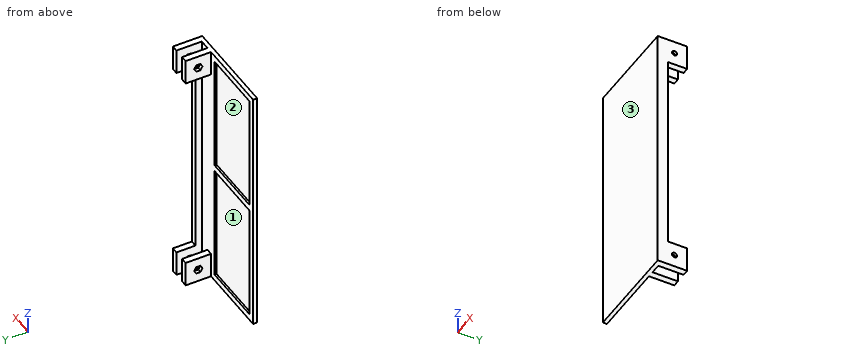
from build123d import *

# Parameters (mm, degrees)
F0_W      = 60
F0_H      = 200
F1_DEPTH  = 3.2
F2_W      = 3
F2_H      = 20
F3_DEPTH  = 20
F5_DEPTH  = 15
F6_DEPTH  = 2
F7_DEPTH  = 2
F8_R      = 2
F9_DEPTH  = 3
F10_DEPTH = 25
F11_R     = 2
F12_DEPTH = 3
F13_DEPTH = 25
F14_W     = 5
F14_H     = 5
F15_DEPTH = 160
F16_W     = 49
F16_H     = 92.5
F17_DEPTH = 1.6


with BuildPart() as f1:
    # F0 (on Front) → F1 (new body)
    with BuildSketch(Plane.XZ):
        with Locations((30, 100)):
            Rectangle(F0_W, F0_H)
    extrude(amount=F1_DEPTH)

    # F2 (on face) → F3 (join)
    with BuildSketch(Plane(origin=(0, 0, 0), x_dir=(-1, 0, 0), z_dir=(0, 1, 0))):
        with Locations((-58.5, 190)):
            Rectangle(F2_W, F2_H)
        with Locations((-58.5, 10)):
            Rectangle(F2_W, F2_H)
        with Locations((-47.5, 190)):
            Rectangle(F2_W, F2_H)
        with Locations((-47.5, 10)):
            Rectangle(F2_W, F2_H)
    extrude(amount=F3_DEPTH)

    # F5 (add): a face of the model
    f5_faces = [f1.faces().sort_by_distance(p)[0] for p in [
        (0, -1.6, 100),
    ]]
    extrude(f5_faces, amount=F5_DEPTH)

    # F6 (add): a face of the model
    f6_faces = [f1.faces().sort_by_distance(p)[0] for p in [
        (60, -1.186588964, 100),
    ]]
    extrude(f6_faces, amount=F6_DEPTH)

    # F7 (add): faces of the model
    f7_faces = [f1.faces().sort_by_distance(p)[0] for p in [
        (46, 10, 190),
        (46, 10, 10),
    ]]
    extrude(f7_faces, amount=F7_DEPTH)

    # F8 (on face) → F9 (cut)
    with BuildSketch(Plane(origin=(57, 0, 0), x_dir=(0, -1, 0), z_dir=(-1, 0, 0))):
        Polygon((-6.7091034656, 10), (-8.3545517328, 12.85), (-11.6454482672, 12.85), (-13.2908965344, 10), (-11.6454482672, 7.15), (-8.3545517328, 7.15), align=None)
        with Locations((-10, 10)):
            Circle(F8_R, mode=Mode.SUBTRACT)
        Polygon((-11.6454482672, 187.15), (-8.3545517328, 187.15), (-6.7091034656, 190), (-8.3545517328, 192.85), (-11.6454482672, 192.85), (-13.2908965344, 190), align=None)
        with Locations((-10, 190)):
            Circle(F8_R, mode=Mode.SUBTRACT)
    extrude(amount=-F9_DEPTH, mode=Mode.SUBTRACT)

    # F10 (cut): faces of the model
    f10_faces = [f1.faces().sort_by_distance(p)[0] for p in [
        (57, 10, 10),
        (57, 10, 190),
    ]]
    extrude(f10_faces, amount=-F10_DEPTH, mode=Mode.SUBTRACT)

    # F11 (on face) → F12 (cut)
    with BuildSketch(Plane(origin=(44, 0, 0), x_dir=(0, -1, 0), z_dir=(-1, 0, 0))):
        Polygon((-6.7091034656, 10), (-8.3545517328, 12.85), (-11.6454482672, 12.85), (-13.2908965344, 10), (-11.6454482672, 7.15), (-8.3545517328, 7.15), align=None)
        with Locations((-10, 10)):
            Circle(F11_R, mode=Mode.SUBTRACT)
        Polygon((-11.6454482672, 187.15), (-8.3545517328, 187.15), (-6.7091034656, 190), (-8.3545517328, 192.85), (-11.6454482672, 192.85), (-13.2908965344, 190), align=None)
        with Locations((-10, 190)):
            Circle(F11_R, mode=Mode.SUBTRACT)
    extrude(amount=-F12_DEPTH, mode=Mode.SUBTRACT)

    # F13 (cut): faces of the model
    f13_faces = [f1.faces().sort_by_distance(p)[0] for p in [
        (44, 10, 190),
        (44, 10, 10),
    ]]
    extrude(f13_faces, amount=-F13_DEPTH, mode=Mode.SUBTRACT)

    # F14 (on face) → F15 (join, through all)
    with BuildSketch(Plane(origin=(0, 0, 180), x_dir=(1, 0, 0), z_dir=(0, 0, -1))):
        with Locations((59.5, -2.5)):
            Rectangle(F14_W, F14_H)
    extrude(amount=F15_DEPTH)

    # F16 (on face) → F17 (cut)
    with BuildSketch(Plane(origin=(0, 0, 0), x_dir=(-1, 0, 0), z_dir=(0, 1, 0))):
        with Locations((-14.5, 51.25)):
            Rectangle(F16_W, F16_H)
        with Locations((-14.5, 148.75)):
            Rectangle(F16_W, F16_H)
    extrude(amount=-F17_DEPTH, mode=Mode.SUBTRACT)


solid = f1.part
Check sheet for the modelled part. Datum: model origin and axes. Units: mm. Face numbers are marked on the shaded views. Give positions to 0.01 mm unless a question says otherwise; leave off trailing zeros. Order: outer loops, then holes, each group sorted by start corner. A loop starts at its lowest first (then second) coordinate and runs counter-clockwise, first axis right, second up. Notation, with made-up numbers: M 31.5,56.25 L 83.5,56.25 A22 ccw 83.5,89.25 Z; hole C 33.25,-23.5 d11. An arc over 180 degrees is marked long. Answer as CSV lines item,"result". Start each with the question number.
Item 1: Cross-section at C-C on x = 54. Enter the section's corners in (y, z).
Item 2: Thickness scan on line 1 (Z direction, x = 47.8, y = 10); line 2 (Z direction, x = 9, y = -0.75); line 3 (Y direction, x = 48.35, z = 190). Record the ranges inside material, lowest first. Write a range as [from, to].
Item 3: Mould release check, pull along X, two halves, no side actions. Record for the marked faces 1, 2 and 3: +X half, -X half, draft (parallel to the pull), parting line (faces both ways), or undercut.
Item 4: Cross-section at A-A on z = 132. Enter the section's corners in (x, y).
Item 5: Cross-section at B-B on x = -5. Enter the section's corners in (y, z).
Item 6: Gauge pin test, flat ends, axial feed: P1, Ø3.5, axis at y = 10, z = 190, coming from the +X side; P2, Ø6, axis at y = 6, z = 194, coming from the -X side; P3, Ø8, axis at x = 46, y = 1.5, coming from the -Z side; P4, Ø5, axis at x = 12, z = 151.5, coming from the +Y side. Record the tip position at first contact, or that the pin passes through.
Established:
1,outline,"M -3.2,0 L 0,0 L 0,200 L -3.2,200 Z"
2,line 1,"z = [0, 8], [12, 20], [180, 188], [192, 200]"
2,line 2,"z = [0, 5], [97.5, 102.5], [195, 200]"
2,line 3,"y = [-3.2, 8], [12, 20]"
3,face 1,"undercut"
3,face 2,"undercut"
3,face 3,"draft"
4,outline,"M -15,-3.2 L 62,-3.2 L 62,5 L 57,5 L 57,0 L 39,0 L 39,-1.6 L -10,-1.6 L -10,0 L -15,0 Z"
5,outline,"M -3.2,0 L 0,0 L 0,5 L -1.6,5 L -1.6,97.5 L 0,97.5 L 0,102.5 L -1.6,102.5 L -1.6,195 L 0,195 L 0,200 L -3.2,200 Z"
6,P1,"passes through"
6,P2,"stops at x = 44"
6,P3,"stops at z = 0"
6,P4,"stops at y = -1.6"
